Geometry: final body of the model. Coordinates: model frame, mm. A direction names the side the tool comes from. Give positions to 0.01 mm unless a question says otherwise; leave off trailing zeros. Loops run counter-clockwise (first coordinate to the right, second up) from the corner with the lowest first, then second, coordinate; pieces in that order, holes last.
```python
from build123d import *

# Parameters (mm, degrees)
F0_W     = 406.4
F0_H     = 406.4
F1_DEPTH = 254
F2_R     = 63.5
F3_DEPTH = 50.8
F4_T     = -25.4


with BuildPart() as f1:
    # F0 (on Top) → F1 (new body)
    with BuildSketch(Plane.XY):
        Rectangle(F0_W, F0_H)
    extrude(amount=F1_DEPTH)

    # F2 (on face) → F3 (join)
    with BuildSketch(Plane.XY.offset(254)):
        with Locations((101.6, 101.6)):
            Circle(F2_R)
        with Locations((101.6, -101.6)):
            Circle(F2_R)
        with Locations((-101.6, -101.6)):
            Circle(F2_R)
        with Locations((-101.6, 101.6)):
            Circle(F2_R)
    extrude(amount=F3_DEPTH)

    # F4
    f4_openings = [f1.faces().sort_by_distance(p)[0] for p in [
        (0, 0, 0),
    ]]
    offset(amount=F4_T, openings=f4_openings, kind=Kind.INTERSECTION)


solid = f1.part
```
Q1. Mould query, pull axis X, two halves, no side actions, for faces 4 (the face through (-102, -101, 279.4)), 5 (the face through (101, 102, 304.8)), 6 (the face through (203.2, -3, 125)). Classes: +X half, -X half, draft (parallel to the pull), parting line (faces both ways), or undercut.
Q2. Material intervals for probe 1 along X at (y, z) = (101.6, 240.5); probe 2 along Y at (x, z) = (-101, 268), sorted ascending.
Q3. Section query A-A, the plane y = -18.5. Return loops of the section in (x, z).
Q4. Reachability of faces 1 (the face through (135.74, 155.14, 279.04)), 2 (the face through (63.537, 103.275, 253.644)), 3 (the face through (101, -101, 304.8)) from +Z, -Z, +X, -X, +Y, -Y: full face, straight path, thin tool, end or side. Return the list, or none.
Q5. Section query C-C, the plane x = -101.6. Return loops of the section in (y, z), and give its area (3 significant figures).
Q6. Section query B-B, the plane z = 84. Return loops of the section in (x, y), and give its area (3 significant figures).
Resolved:
1. face 4: undercut
1. face 5: draft
1. face 6: +X half
2. probe 1: x = -203.2 to -139.7, -63.5 to 63.5, 139.7 to 203.2
2. probe 2: y = -165.1 to -139.7, -63.5 to -38.1, 38.1 to 63.5, 139.7 to 165.1
3. outline: (-203.2, 0) - (-177.8, 0) - (-177.8, 228.6) - (177.8, 228.6) - (177.8, 0) - (203.2, 0) - (203.2, 254) - (-203.2, 254) - close
4. face 1: +Z
4. face 2: -Z
4. face 3: +Z, +X, -X, +Y, -Y
5. outline: (-203.2, 0) - (-177.8, 0) - (-177.8, 228.6) - (-139.7, 228.6) - (-139.7, 279.4) - (-63.5, 279.4) - (-63.5, 228.6) - (63.5, 228.6) - (63.5, 279.4) - (139.7, 279.4) - (139.7, 228.6) - (177.8, 228.6) - (177.8, 0) - (203.2, 0) - (203.2, 254) - (165.1, 254) - (165.1, 304.8) - (38.1, 304.8) - (38.1, 254) - (-38.1, 254) - (-38.1, 304.8) - (-165.1, 304.8) - (-165.1, 254) - (-203.2, 254) - close
5. area: 27,100 mm2
6. outline: (-203.2, -203.2) - (203.2, -203.2) - (203.2, 203.2) - (-203.2, 203.2) - close; hole (-177.8, -177.8) - (177.8, -177.8) - (177.8, 177.8) - (-177.8, 177.8) - close
6. area: 38,700 mm2
